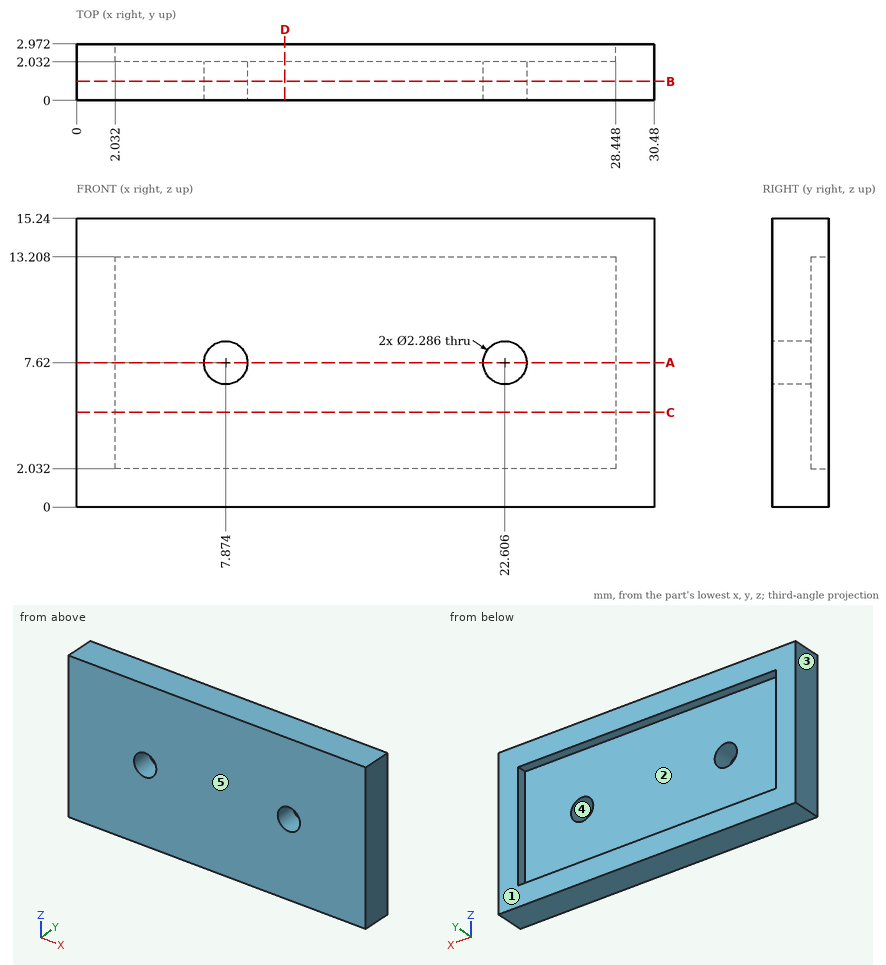
Answer from the drawing. Dimensions are ordinates in mm from the lowest x, y and z of the part. A direction names the side the tool comes from. Coordinates: 2 decimals unless noted, no trailing zeros. Write each loop counter-clockwise with the first axis right and the second up, starting at its lowest first coordinate (ties: lowest second). Pieces come first, ordered by that corner, then holes. Notation, with made-up numbers: M 32.25,50.5 L 41.25,50.5 A26 ccw 41.25,88.5 Z; hole C -11.75,24.25 d2. An arc over 180 degrees is marked long. Use one line per item in the form item = value. Start each with the question number.
1. The part is cut by section B-B (y = 1). Give the vertices of the cut face in (x, z).
2. Straight lines are drawn through the part: probe 1 along X at (y, z) = (0.3, 7.5); probe 2 along X at (y, z) = (0.85, 8.5) (1 decimal); probe 3 along X at (y, z) = (2.6, 6). For each, find the intervals that lie inside material, in ascending order. Write a range as from..to.
3. The part is cut by section D-D (x = 11). Give the vertices of the cut face in (y, z).
4. The part is cut by section C-C (z = 5). Give the vertices of the cut face in (x, y).
5. The mould has two halves that part along X. Classify the marked faces 3, 4 and 5: released by +X, released by -X, zero draft, split by the parting line, or undercut.
6. The part is cut by section A-A (z = 7.62). Give the vertices of the cut face in (x, y).
7. A tool of negligible diameter and unlimited length cuts with its end or side. For the marked faces 1 and 2, from which of +Z, -Z, +X, -X, +Y, -Y can it reach the whole face along a straight path? Write none if from no direction.
Evaluation:
q1.outline = M 0,0 L 30.48,0 L 30.48,15.24 L 0,15.24 Z; hole C 7.87,7.62 d2.29; hole C 22.61,7.62 d2.29
q2.probe_1 = 0..6.74, 9.01..21.47, 23.74..30.48
q2.probe_2 = 0..7.1, 8.6..21.9, 23.3..30.5
q2.probe_3 = 0..2.03, 28.45..30.48
q3.outline = M 0,0 L 2.97,0 L 2.97,2.03 L 2.03,2.03 L 2.03,13.21 L 2.97,13.21 L 2.97,15.24 L 0,15.24 Z
q4.outline = M 0,0 L 30.48,0 L 30.48,2.97 L 28.45,2.97 L 28.45,2.03 L 2.03,2.03 L 2.03,2.97 L 0,2.97 Z
q5.face_3 = released by -X
q5.face_4 = undercut
q5.face_5 = zero draft
q6.outline = M 0,0 L 6.73,0 L 6.73,2.03 L 2.03,2.03 L 2.03,2.97 L 0,2.97 Z; M 9.02,0 L 21.46,0 L 21.46,2.03 L 9.02,2.03 Z; M 23.75,0 L 30.48,0 L 30.48,2.97 L 28.45,2.97 L 28.45,2.03 L 23.75,2.03 Z
q7.face_1 = +Z, -Z, +X, -X, +Y
q7.face_2 = +Y
